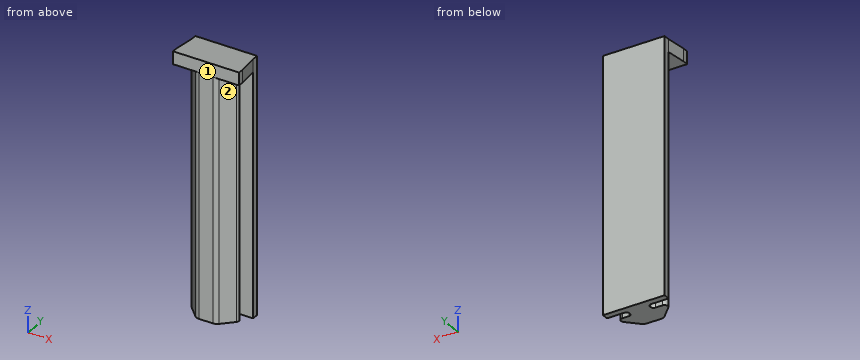
from build123d import *

# Parameters (mm, degrees)
BOSS_EXTRUDE1_DEPTH = 76.2
BOSS_EXTRUDE2_START = 4
BOSS_EXTRUDE2_DEPTH = 4


with BuildPart() as part:
    # Sketch1 → Boss-Extrude1 (new body)
    with BuildSketch(Plane.XY):
        with BuildLine():
            Line((-6.348478019, 10.4902), (-4.190365, 10.4902))
            ThreePointArc((-4.190365, 10.4902), (-3.52627506, 10.76527506), (-3.2512, 11.429365))
            Line((-3.2512, 11.429365), (-3.2512, 11.760835))
            ThreePointArc((-3.2512, 11.760835), (-3.52627506, 12.42492494), (-4.190365, 12.7))
            Line((-4.190365, 12.7), (-5.243578019, 12.7))
            Line((-5.243578019, 12.7), (-9.803703152, 12.7))
            Line((-9.803703152, 12.7), (-9.803703152, 14.7))
            Line((-9.803703152, 14.7), (9.803703152, 14.7))
            Line((9.803703152, 14.7), (9.803703152, 12.7))
            Line((9.803703152, 12.7), (6.348478019, 12.7))
            Line((6.348478019, 12.7), (5.243578019, 12.7))
            Line((5.243578019, 12.7), (4.190365, 12.7))
            ThreePointArc((4.190365, 12.7), (3.52627506, 12.42492494), (3.2512, 11.760835))
            Line((3.2512, 11.760835), (3.2512, 11.429365))
            ThreePointArc((3.2512, 11.429365), (3.52627506, 10.76527506), (4.190365, 10.4902))
            Line((4.190365, 10.4902), (6.348478019, 10.4902))
            ThreePointArc((6.348478019, 10.4902), (7.335478831, 9.830707141), (7.103895736, 8.666460301))
            Line((7.103895736, 8.666460301), (3.737334563, 5.299899128))
            ThreePointArc((3.737334563, 5.299899128), (3.015479634, 4.817571085), (2.16399369, 4.6482))
            Line((2.16399369, 4.6482), (-2.16399369, 4.6482))
            ThreePointArc((-2.16399369, 4.6482), (-3.015479634, 4.817571085), (-3.737334563, 5.299899128))
            Line((-3.737334563, 5.299899128), (-7.103895736, 8.666460301))
            ThreePointArc((-7.103895736, 8.666460301), (-7.335478831, 9.830707141), (-6.348478019, 10.4902))
        make_face()
    extrude(amount=-BOSS_EXTRUDE1_DEPTH)

    # Sketch1_3 → Boss-Extrude2 (add)
    with BuildSketch(Plane.XY.offset(BOSS_EXTRUDE2_START)):
        with BuildLine():
            ThreePointArc((-4.190365, 10.4902), (-3.52627506, 10.76527506), (-3.2512, 11.429365))
            Line((-3.2512, 11.429365), (-3.2512, 11.760835))
            ThreePointArc((-3.2512, 11.760835), (-3.52627506, 12.42492494), (-4.190365, 12.7))
            Line((-4.190365, 12.7), (-5.243578019, 12.7))
            Line((-5.243578019, 12.7), (-9.803703152, 12.7))
            Line((-9.803703152, 12.7), (-10.4902, 6.348478019))
            Line((-10.4902, 6.348478019), (-10.4902, 4.6482))
            Line((-10.4902, 4.6482), (-2.16399369, 4.6482))
            ThreePointArc((-2.16399369, 4.6482), (-3.015479634, 4.817571085), (-3.737334563, 5.299899128))
            Line((-3.737334563, 5.299899128), (-7.103895736, 8.666460301))
            ThreePointArc((-7.103895736, 8.666460301), (-7.335478831, 9.830707141), (-6.348478019, 10.4902))
            Line((-6.348478019, 10.4902), (-4.190365, 10.4902))
        make_face()
        with BuildLine():
            Line((-6.348478019, 10.4902), (-4.190365, 10.4902))
            ThreePointArc((-4.190365, 10.4902), (-3.52627506, 10.76527506), (-3.2512, 11.429365))
            Line((-3.2512, 11.429365), (-3.2512, 11.760835))
            ThreePointArc((-3.2512, 11.760835), (-3.52627506, 12.42492494), (-4.190365, 12.7))
            Line((-4.190365, 12.7), (-5.243578019, 12.7))
            Line((-5.243578019, 12.7), (-9.803703152, 12.7))
            Line((-9.803703152, 12.7), (-9.803703152, 14.7))
            Line((-9.803703152, 14.7), (9.803703152, 14.7))
            Line((9.803703152, 14.7), (9.803703152, 12.7))
            Line((9.803703152, 12.7), (6.348478019, 12.7))
            Line((6.348478019, 12.7), (5.243578019, 12.7))
            Line((5.243578019, 12.7), (4.190365, 12.7))
            ThreePointArc((4.190365, 12.7), (3.52627506, 12.42492494), (3.2512, 11.760835))
            Line((3.2512, 11.760835), (3.2512, 11.429365))
            ThreePointArc((3.2512, 11.429365), (3.52627506, 10.76527506), (4.190365, 10.4902))
            Line((4.190365, 10.4902), (6.348478019, 10.4902))
            ThreePointArc((6.348478019, 10.4902), (7.335478831, 9.830707141), (7.103895736, 8.666460301))
            Line((7.103895736, 8.666460301), (3.737334563, 5.299899128))
            ThreePointArc((3.737334563, 5.299899128), (3.015479634, 4.817571085), (2.16399369, 4.6482))
            Line((2.16399369, 4.6482), (-2.16399369, 4.6482))
            ThreePointArc((-2.16399369, 4.6482), (-3.015479634, 4.817571085), (-3.737334563, 5.299899128))
            Line((-3.737334563, 5.299899128), (-7.103895736, 8.666460301))
            ThreePointArc((-7.103895736, 8.666460301), (-7.335478831, 9.830707141), (-6.348478019, 10.4902))
        make_face()
        with BuildLine():
            ThreePointArc((3.737334563, 5.299899128), (3.015479634, 4.817571085), (2.16399369, 4.6482))
            Line((2.16399369, 4.6482), (10.4902, 4.6482))
            Line((10.4902, 4.6482), (10.4902, 6.348478019))
            Line((10.4902, 6.348478019), (9.803703152, 12.7))
            Line((9.803703152, 12.7), (6.348478019, 12.7))
            Line((6.348478019, 12.7), (5.243578019, 12.7))
            Line((5.243578019, 12.7), (4.190365, 12.7))
            ThreePointArc((4.190365, 12.7), (3.52627506, 12.42492494), (3.2512, 11.760835))
            Line((3.2512, 11.760835), (3.2512, 11.429365))
            ThreePointArc((3.2512, 11.429365), (3.52627506, 10.76527506), (4.190365, 10.4902))
            Line((4.190365, 10.4902), (6.348478019, 10.4902))
            ThreePointArc((6.348478019, 10.4902), (7.335478831, 9.830707141), (7.103895736, 8.666460301))
            Line((7.103895736, 8.666460301), (3.737334563, 5.299899128))
        make_face()
    extrude(amount=-BOSS_EXTRUDE2_DEPTH)


solid = part.part
Input: part model. Units: mm. Frame: model coordinates. Face numbers are marked on the shaded views. A direction names the side the tool comes from. Coordinates: 2 decimals unless noted, no trailing zeros. Write each loop counter-clockwise with the first axis right and the second up, starting at its lowest first coordinate (ties: lowest second). Pieces come first, ordered by that corner, then holes. Notation, with made-up numbers: M 15.25,50.25 L 20.25,50.25 A21 cw 20.25,81.25 Z; hole C 60,88 d9. An arc over 180 degrees is marked long. Answer as a JSON object with one key per item and string values. Group by question number.
(1) Section A-A on z = -60. Output: boundary loops of the cut face in (x, y), plus the area to 3 significant figures.
(2) Section C-C on y = 9.5. Output: boundary loops of the cut face in (x, z), plus the area to 3 significant figures.
(3) Contact query for flat-ended pins moving along their axis: P1, Ø1.6, axis at y = 13.5, z = -23.5, coming from the -X side; P2, Ø2, axis at y = 8, z = -20, coming from the -X side; P3, Ø1.7, axis at x = 6, z = -52.5, coming from the -Y side. Output: stop coordinate, or through.
(4) Ray query, line 1 along Z through (x, y) = (7, 11); line 2 along X through (y, z) = (9.5, -60.5); line 3 along Y through (x, z) = (-4, -68.5). Return the intervals inside material, ascending. Write a range as [from, to].
(5) Set-up query: the marked faces 1 and 2. Return all of +Z, -Z, +X, -X, +Y, -Y with unobstructed straight access to the full face (end or side cutting, diameter ignored); none if empty.
(6) Section B-B on x = 5.25. Output: boundary loops of the cut face in (y, z), plus the area to 3 significant figures.
Result set:
{
 "1": {"outline": "M -9.8,12.7 L -4.19,12.7 A0.94 cw -3.25,11.76 L -3.25,11.43 A0.94 cw -4.19,10.49 L -6.35,10.49 A1.07 ccw -7.1,8.67 L -3.74,5.3 A2.23 ccw -2.16,4.65 L 2.16,4.65 A2.23 ccw 3.74,5.3 L 7.1,8.67 A1.07 ccw 6.35,10.49 L 4.19,10.49 A0.94 cw 3.25,11.43 L 3.25,11.76 A0.94 cw 4.19,12.7 L 9.8,12.7 L 9.8,14.7 L -9.8,14.7 Z", "area": "121 mm2"},
 "2": {"outline": "M -10.15,0 L -7.41,0 L -7.41,-76.2 L 7.41,-76.2 L 7.41,0 L 10.15,0 L 10.15,4 L -10.15,4 Z", "area": "1,210 mm2"},
 "3": {"P1": "stops at x = -9.8", "P2": "stops at x = -7.33", "P3": "stops at y = 6.71"},
 "4": {"line 1": "z = [0, 4]", "line 2": "x = [-7.41, 7.41]", "line 3": "y = [5.56, 10.51], [12.68, 14.7]"},
 "5": {"face 1": "+Z, -Z, +X, -X, -Y", "face 2": "-Z, +X, -Y"},
 "6": {"outline": "M 4.65,0 L 6.81,0 L 6.81,-76.2 L 10.49,-76.2 L 10.49,0 L 12.7,0 L 12.7,-76.2 L 14.7,-76.2 L 14.7,4 L 4.65,4 Z", "area": "473 mm2"}
}
